Read the model definition and answer for the solid it produces. Units are mm, in the model's axes. A direction names the side the tool comes from. Give positions to 0.01 mm unless a question says otherwise; leave off trailing zeros. Order: outer loops, then holes, each group sorted by start corner. A loop starts at its lowest first (then second) coordinate and runs counter-clockwise, first axis right, second up.
```python
from build123d import *

# Parameters (mm, degrees)
PARTS_W             = 29.2
PARTS_H             = 21.15
MAIN_FACE_DEPTH     = 2
SKETCH3_R           = 2.525
IR_CUT_DEPTH        = 2
TSOP_GROOVE_DEPTH   = 1.5
SKETCH4_W           = 5.4
SKETCH4_H           = 3.4
TOF_CUT_DEPTH       = 2
SKETCH6_R           = 1.575
SHAFTS_DEPTH        = 5
CHAMFER1_SIZE       = 0.2
SKETCH7_W           = 15
SKETCH7_H           = 3.5
PINSLOTS_DEPTH      = 1
TOFWINDOW_SIZE      = 1
SKETCH8_W           = 1.5
SKETCH8_H           = 6
BOSS_EXTRUDE1_DEPTH = 6
SKETCH14_W          = 1.5
SKETCH14_H          = 4
BOSS_EXTRUDE4_DEPTH = 5
SKETCH15_W          = 24.8
SKETCH15_H          = 4
BOSS_EXTRUDE5_DEPTH = 2
CUT_EXTRUDE4_REACH  = 31.332
SKETCH16_R          = 1
CUT_EXTRUDE5_START  = -0.5
CUT_EXTRUDE5_DEPTH  = 0.5
FILLET1_R           = 0.5


with BuildPart() as part:
    # Parts → Main Face (new body)
    with BuildSketch(Plane(origin=(0, 0, 0), x_dir=(1, 0, 0), z_dir=(0, 1, 0))):
        with Locations((0, 3.175)):
            Rectangle(PARTS_W, PARTS_H)
    extrude(amount=-MAIN_FACE_DEPTH)

    # Sketch3 → IR Cut (cut)
    with BuildSketch(Plane(origin=(0, 0, 0), x_dir=(1, 0, 0), z_dir=(0, 1, 0))):
        with Locations(Location((7.3875, 9.075, 0), (0, 0, 270))):
            Circle(SKETCH3_R)
        Polygon((-2.6125, 11.75), (-2.6125, 6.4), (-9.4125, 6.4), (-9.4125, 5.9), (-9.9125, 5.9), (-9.9125, 6.4), (-9.9125, 11.75), (-9.9125, 12.25), (-9.4125, 12.25), (-9.4125, 11.75), align=None)
    extrude(amount=-IR_CUT_DEPTH, mode=Mode.SUBTRACT)

    # Sketch5 → TSOP Groove (cut)
    with BuildSketch(Plane.XZ.offset(2)):
        Polygon((-2.6125, -11.75), (-2.6125, -6.4), (-2.6125, -5.9), (1.3875, -5.9), (1.3875, -6.4), (1.3875, -11.75), (1.3875, -12.25), (-2.6125, -12.25), align=None)
    extrude(amount=-TSOP_GROOVE_DEPTH, mode=Mode.SUBTRACT)

    # Sketch4 → TOF Cut (cut)
    with BuildSketch(Plane(origin=(0, 0, 0), x_dir=(1, 0, 0), z_dir=(0, 1, 0))):
        with Locations((0, 1.6)):
            Rectangle(SKETCH4_W, SKETCH4_H)
    extrude(amount=-TOF_CUT_DEPTH, mode=Mode.SUBTRACT)

    # Sketch6 → Shafts (add)
    with BuildSketch(Plane.XZ.offset(2)):
        with Locations(Location((-9.9, 0, 0), (0, 0, 270))):
            Circle(SKETCH6_R)
        with Locations(Location((9.9, 0, 0), (0, 0, 270))):
            Circle(SKETCH6_R)
    extrude(amount=SHAFTS_DEPTH)

    # Chamfer1
    chamfer1_edges = [part.edges().sort_by_distance(p)[0] for p in [
        (9.9, -7, 1.575),
        (-9.9, -7, 1.575),
    ]]
    chamfer(chamfer1_edges, length=CHAMFER1_SIZE)

    # Sketch7 → PinSlots (cut)
    with BuildSketch(Plane.XZ.offset(2)):
        with Locations((0, 3.15)):
            Rectangle(SKETCH7_W, SKETCH7_H)
    extrude(amount=-PINSLOTS_DEPTH, mode=Mode.SUBTRACT)

    # ToFWindow
    tofwindow_edges = [part.edges().sort_by_distance(p)[0] for p in [
        (-2.7, 0, -1.6),
        (0, 0, 0.1),
        (2.7, 0, -1.6),
        (0, 0, -3.3),
    ]]
    chamfer(tofwindow_edges, length=TOFWINDOW_SIZE)

    # Sketch8 → Boss-Extrude1 (add)
    with BuildSketch(Plane.XZ.offset(2)):
        with Locations((-11.65, -8.75)):
            Rectangle(SKETCH8_W, SKETCH8_H)
        with Locations((11.65, -8.75)):
            Rectangle(SKETCH8_W, SKETCH8_H)
    extrude(amount=BOSS_EXTRUDE1_DEPTH)

    # Sketch14 → Boss-Extrude4 (add)
    with BuildSketch(Plane(origin=(0, 0, -11.75), x_dir=(-1, 0, 0), z_dir=(0, 0, -1))):
        with Locations((-11.65, -6)):
            Rectangle(SKETCH14_W, SKETCH14_H)
        with Locations((11.65, -6)):
            Rectangle(SKETCH14_W, SKETCH14_H)
    extrude(amount=BOSS_EXTRUDE4_DEPTH)

    # Sketch15 → Boss-Extrude5 (add)
    with BuildSketch(Plane(origin=(0, 0, -16.75), x_dir=(-1, 0, 0), z_dir=(0, 0, -1))):
        with Locations((0, -6)):
            Rectangle(SKETCH15_W, SKETCH15_H)
    extrude(amount=BOSS_EXTRUDE5_DEPTH)

    # Sketch16 → Cut-Extrude4 (cut, up to next)
    with BuildSketch(Plane.XY.offset(-16.75), mode=Mode.PRIVATE) as cut_extrude4_sk1:
        with Locations((-4.5, -6)):
            Circle(SKETCH16_R)
    cut_extrude4_tool1 = extrude(cut_extrude4_sk1.sketch, amount=-CUT_EXTRUDE4_REACH, mode=Mode.PRIVATE) & part.part
    # Sketch16 → Cut-Extrude4 (cut, up to next)
    with BuildSketch(Plane.XY.offset(-16.75), mode=Mode.PRIVATE) as cut_extrude4_sk2:
        with Locations((-1.5, -6)):
            Circle(SKETCH16_R)
    cut_extrude4_tool2 = extrude(cut_extrude4_sk2.sketch, amount=-CUT_EXTRUDE4_REACH, mode=Mode.PRIVATE) & part.part
    # Sketch16 → Cut-Extrude4 (cut, up to next)
    with BuildSketch(Plane.XY.offset(-16.75), mode=Mode.PRIVATE) as cut_extrude4_sk3:
        with Locations(Location((1.5, -6, 0), (0, 0, 180))):
            Circle(SKETCH16_R)
    cut_extrude4_tool3 = extrude(cut_extrude4_sk3.sketch, amount=-CUT_EXTRUDE4_REACH, mode=Mode.PRIVATE) & part.part
    # Sketch16 → Cut-Extrude4 (cut, up to next)
    with BuildSketch(Plane.XY.offset(-16.75), mode=Mode.PRIVATE) as cut_extrude4_sk4:
        with Locations(Location((4.5, -6, 0), (0, 0, 180))):
            Circle(SKETCH16_R)
    cut_extrude4_tool4 = extrude(cut_extrude4_sk4.sketch, amount=-CUT_EXTRUDE4_REACH, mode=Mode.PRIVATE) & part.part
    add(cut_extrude4_tool1.solids().sort_by_distance((-4.5, -6, -16.75))[0], mode=Mode.SUBTRACT)
    add(cut_extrude4_tool2.solids().sort_by_distance((-1.5, -6, -16.75))[0], mode=Mode.SUBTRACT)
    add(cut_extrude4_tool3.solids().sort_by_distance((1.5, -6, -16.75))[0], mode=Mode.SUBTRACT)
    add(cut_extrude4_tool4.solids().sort_by_distance((4.5, -6, -16.75))[0], mode=Mode.SUBTRACT)

    # Sketch17 → Cut-Extrude5 (cut)
    with BuildSketch(Plane(origin=(0, 0, -18.75), x_dir=(-1, 0, 0), z_dir=(0, 0, -1)).offset(CUT_EXTRUDE5_START)):
        with BuildLine():
            Line((-5, -6.866025404), (-5, -8))
            Line((-5, -8), (-4, -8))
            Line((-4, -8), (-4, -6.866025404))
            ThreePointArc((-4, -6.866025404), (-4.5, -7), (-5, -6.866025404))
        make_face()
        with BuildLine():
            Line((-1, -8), (-1, -6.866025404))
            ThreePointArc((-1, -6.866025404), (-1.5, -7), (-2, -6.866025404))
            Line((-2, -6.866025404), (-2, -8))
            Line((-2, -8), (-1, -8))
        make_face()
        with BuildLine():
            Line((2, -8), (2, -6.866025404))
            ThreePointArc((2, -6.866025404), (1.5, -7), (1, -6.866025404))
            Line((1, -6.866025404), (1, -8))
            Line((1, -8), (2, -8))
        make_face()
        with BuildLine():
            Line((5, -8), (5, -6.866025404))
            ThreePointArc((5, -6.866025404), (4.5, -7), (4, -6.866025404))
            Line((4, -6.866025404), (4, -8))
            Line((4, -8), (5, -8))
        make_face()
    extrude(amount=CUT_EXTRUDE5_DEPTH, mode=Mode.SUBTRACT)

    # Fillet1
    fillet1_edges = [part.edges().sort_by_distance(p)[0] for p in [
        (-5, -7.433012702, -18.25),
        (-4, -7.433012702, -18.25),
        (-2, -7.433012702, -18.25),
        (-1, -7.433012702, -18.25),
        (1, -7.433012702, -18.25),
        (2, -7.433012702, -18.25),
        (4, -7.433012702, -18.25),
        (5, -7.433012702, -18.25),
    ]]
    fillet(fillet1_edges, radius=FILLET1_R - 0.0001)  # a hair under: the kernel refuses the full size


solid = part.part
```
1) The part is cut by section C-C on z = -9.75. Determine the outline of the cut face in (x, y).
Final values:
outline: (-14.6, -2) - (-12.4, -2) - (-12.4, -8) - (-10.9, -8) - (-10.9, -2) - (-9.91, -2) - (-9.91, 0) - (-14.6, 0) - close; (-2.61, -0.5) - (1.39, -0.5) - (1.39, -2) - (4.95, -2) - (4.95, 0) - (-2.61, 0) - close; (9.82, -2) - (10.9, -2) - (10.9, -8) - (12.4, -8) - (12.4, -2) - (14.6, -2) - (14.6, 0) - (9.82, 0) - close
2) The part is cut by section B-B on y = -4.5. Determine the outline of the cut face in (x, z) (3 decimals), and give its area (3 significant figures).
Final values:
outline: (-12.4, -18.75) - (12.4, -18.75) - (12.4, -5.75) - (10.9, -5.75) - (10.9, -16.75) - (-10.9, -16.75) - (-10.9, -5.75) - (-12.4, -5.75) - close; circle Ø3.15 at (-9.9, 0); circle Ø3.15 at (9.9, 0)
area: 98.2 mm2
3) Consider L1, parallel to X at y = -6, z = -17.5; L2, parallel to X at y = -6.75, z = 0 (3 decimals); L3, parallel to Z at x = -2, y = -1.25. Determine where each line is inside the solid, lowest interval first.
Final values:
L1: x = -12.4 to -5.5, -3.5 to -2.5, -0.5 to 0.5, 2.5 to 3.5, 5.5 to 12.4
L2: x = -11.475 to -8.325, 8.325 to 11.475
L3: z = -13.75 to -12.25, -5.9 to -3.3, 0.1 to 1.4, 4.9 to 7.4
4) The part is cut by section A-A on z = -2. Determine the outline of the cut face in (x, y), and give its area (3 significant figures).
Final values:
outline: (-14.6, -2) - (-2.7, -2) - (-2.7, -1) - (-3.7, 0) - (-14.6, 0) - close; (2.7, -2) - (14.6, -2) - (14.6, 0) - (3.7, 0) - (2.7, -1) - close
area: 46.6 mm2
5) Given pin 1 (1.8 mm diameter, centred on x = 3, z = 2.5, fed in from -Y); pin 2 (1 mm diameter, centred on x = 10, z = -9, fed in from -Y); pin 3 (3 mm diameter, centred on y = -6.5, z = -12, fed in from +X); pin 4 (1.2 mm diameter, centred on x = -4.5, y = -6, fed in from -Z), each flat-ended and moving along its own axis, determine where each tip first touches the part or whether it passes through.
Final values:
pin 1: stops at y = -1
pin 2: stops at y = -2
pin 3: stops at x = 12.4
pin 4: passes through
6) A tool of negligible diameter and unlimited length cuts with its end or side. For faces 4 (the face through (10, -7, 0)), 5 (the face through (-12, -5, -5.75)), 6 (the face through (-8.34, -4.37, 0.21)), 7 (the face through (12.4, -6, -12)), 8 (the face through (-12.4, -6, -12)), from which of +Z, -Z, +X, -X, +Y, -Y can it reach the whole face along a straight path? Write none if from no direction.
Final values:
face 4: +Z, +X, -X, -Y
face 5: +X, -X, -Y
face 6: -Y
face 7: +Z, -Z, +X, -Y
face 8: +Z, -Z, -X, -Y
7) For a pull along Z with two mould halves and no side action, classify faces 1 (the face through (4.717, -5.024, -17.736)), 2 (the face through (12, -3, -11.75)), 3 (the face through (-1, -1, -12.25)) as released by +Z, released by -Z, zero draft, split by the parting line, or undercut.
Final values:
face 1: zero draft
face 2: released by -Z
face 3: undercut
8) The part is cut by section D-D on y = -2.75. Determine the outline of the cut face in (x, z) (3 decimals).
Final values:
outline: (-12.4, -11.75) - (-10.9, -11.75) - (-10.9, -5.75) - (-12.4, -5.75) - close; circle Ø3.15 at (-9.9, 0); circle Ø3.15 at (9.9, 0); (10.9, -11.75) - (12.4, -11.75) - (12.4, -5.75) - (10.9, -5.75) - close
